Verification items for the finished model (mm, model axes). A direction names the side the tool comes from. Coordinates: 2 decimals unless noted, no trailing zeros. Loops run counter-clockwise (first coordinate to the right, second up) from the corner with the lowest first, then second, coordinate; pieces in that order, holes last. Notation, with made-up numbers: (66.5, 87.25) - (76.5, 87.25) arc R20 cw to (76.5, 93.25) - close; hole circle Ø3 at (27, -36.75). An arc over 180 degrees is marked (long way). Answer as CSV lines item,"result". Start each with the question number.
1. Set-up check for faces 1 (the flat face through (1, 5, 14)), 2 (the flat face through (-5.3, 0, 9)), 3 (the flat face through (0, 5.262, 15)), 4 (the flat face through (-4, 3.75, 13)): record each of +Z, -Z, +X, -X, +Y, -Y from which the full face is reachable in a straight line by a thin tool's end or side.
2. Cross-section at C-C (z = 17). Enter the section's corners in (x, y).
3. Gauge pin test, flat ends, axial feed: P1, Ø1, axis at x = 4.5, z = 15, coming from the +Y side; P2, Ø1.4, axis at y = 5, z = 11, coming from the +X side; P3, Ø4, axis at y = 0, z = 15, coming from the -X side. Record the tip position at first contact, or that the pin passes through.
4. Material ranges on line 1 (X direction, y = 0.5, z = 11); line 2 (Y direction, x = -2.5, z = 16.5); line 3 (Y direction, x = 0.5, z = 11), recorded low to high. Write a range as [from, to].
5. Cross-section at A-A (y = 1). Enter the section's corners in (x, z).
6. Cross-section at B-B (x = 0.5). Enter the section's corners in (y, z).
7. Cross-section at D-D (z = 5.25). Enter the section's corners in (x, y).
```python
from build123d import *

# Parameters (mm, degrees)
F0_W        = 10.6
F0_H        = 5.5
F0_W_2      = 2
F0_H_2      = 1.512365222
F1_DEPTH    = 19
F0_W_3      = 16.5
F0_H_3      = 12
F2_DEPTH    = 8
F3_R        = 2
F4_T4_DEPTH = 2


# Not quite as in the source:
# - a fillet or chamfer that OpenCascade refuses, or shapes differently, is made with other operations: its cross-section is extruded or revolved along the edge and cut away or added


with BuildPart() as f1:
    # F0 (on Top) → F1 (new body)
    with BuildSketch(Plane.XY):
        Polygon((-6.3, -3.75), (6.3, -3.75), (6.3, 3.75), (1, 3.75), (-1, 3.75), (-6.3, 3.75), align=None)
        Rectangle(F0_W, F0_H, mode=Mode.SUBTRACT)
        with Locations((0, 4.506182611)):
            Rectangle(F0_W_2, F0_H_2)
    extrude(amount=F1_DEPTH)

    # F0 (on Top) → F2 (join)
    with BuildSketch(Plane.XY):
        with Locations((0, 0.5489425384)):
            Rectangle(F0_W_3, F0_H_3)
        Polygon((6.3, 3.75), (6.3, -3.75), (-6.3, -3.75), (-6.3, 3.75), (-1, 3.75), (-1, 5.262365222), (1, 5.262365222), (1, 3.75), align=None, mode=Mode.SUBTRACT)
    extrude(amount=F2_DEPTH)

    # F3
    f3_edges = [f1.edges().sort_by_distance(p)[0] for p in [
        (-8.25, -5.451057, 4),
        (8.25, -5.451057, 4),
        (8.25, 6.548943, 4),
        (-8.25, 6.548943, 4),
    ]]
    fillet(f3_edges, radius=F3_R)

    # F4: chamfer of 3 x 1.4 on 1 edges, made by hand


with BuildPart() as f4_tool2:
    # F4_s3 → F4_t4 (new body)
    with BuildSketch(Plane.YZ.offset(-1)):
        Polygon((6.662365222, 8), (5.262365222, 11), (5.262365222, 8), align=None)
    extrude(amount=F4_T4_DEPTH)

    split(bisect_by=Plane.XZ.offset(-6.5489425384), keep=Keep.TOP)


with BuildPart() as f1_1:
    add(f1.part)

    # F4_t1: union F4_tool2
    add(f4_tool2.part)


solid = f1_1.part
```
Values follow:
1,face 1,"+Z, +X, +Y"
1,face 2,"+Z, -Z"
1,face 3,"+Z, +X, -X, +Y"
1,face 4,"+Z, -X, +Y"
2,outline,"(-6.3, -3.75) - (6.3, -3.75) - (6.3, 3.75) - (1, 3.75) - (1, 5.26) - (-1, 5.26) - (-1, 3.75) - (-6.3, 3.75) - close; hole (-5.3, -2.75) - (5.3, -2.75) - (5.3, 2.75) - (-5.3, 2.75) - close"
3,P1,"stops at y = 3.75"
3,P2,"stops at x = 1"
3,P3,"stops at x = -6.3"
4,line 1,"x = [-6.3, -5.3], [5.3, 6.3]"
4,line 2,"y = [-3.75, -2.75], [2.75, 3.75]"
4,line 3,"y = [-3.75, -2.75], [2.75, 5.26]"
5,outline,"(-8.25, 0) - (-5.3, 0) - (-5.3, 19) - (-6.3, 19) - (-6.3, 8) - (-8.25, 8) - close; (5.3, 0) - (8.25, 0) - (8.25, 8) - (6.3, 8) - (6.3, 19) - (5.3, 19) - close"
6,outline,"(-5.45, 0) - (-2.75, 0) - (-2.75, 19) - (-3.75, 19) - (-3.75, 8) - (-5.45, 8) - close; (2.75, 0) - (6.55, 0) - (6.55, 8.24) - (5.26, 11) - (5.26, 19) - (2.75, 19) - close"
7,outline,"(-8.25, -3.45) arc R2 ccw to (-6.25, -5.45) - (6.25, -5.45) arc R2 ccw to (8.25, -3.45) - (8.25, 4.55) arc R2 ccw to (6.25, 6.55) - (-6.25, 6.55) arc R2 ccw to (-8.25, 4.55) - close; hole (-5.3, -2.75) - (5.3, -2.75) - (5.3, 2.75) - (-5.3, 2.75) - close"
